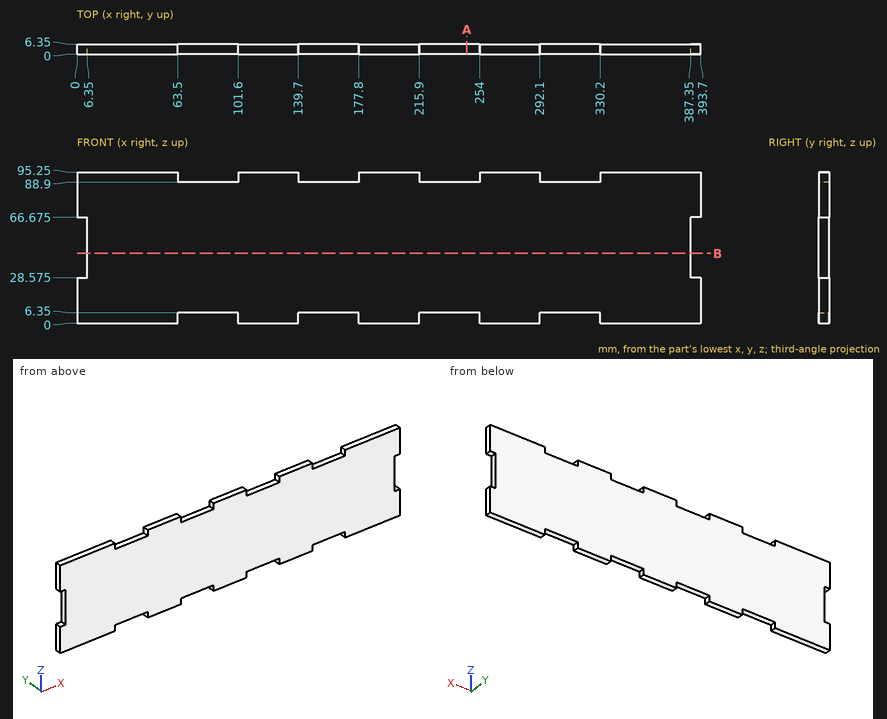
Verification items for this drawing (mm, ordinates from the low corner). Give positions to 0.01 mm unless a question says otherwise; leave off trailing zeros. Loops run counter-clockwise (first coordinate to the right, second up) from the corner with the lowest first, then second, coordinate; pieces in that order, holes last. Notation, with made-up numbers: M 19,49.25 L 69,49.25 A28 ccw 69,74.25 Z; hole C -31.75,31 d1. An arc over 180 degrees is marked long. Return JSON: item names as keys, results as strings. Group by question number.
1. Cross-section at B-B on z = 44. Record the boundary of the cut face in (x, y), plus the area to 3 significant figures.
2. Go/stop test with flat-tipped pins: pin 1 (3 mm diameter, centred on x = 316, y = 3, fed in from +Z); pin 2 (2 mm diameter, centred on y = 4.5, z = 56.5, fed in from +X); pin 3 (3 mm diameter, centred on x = 167, y = 3, fed in from -Z). Record where each tip stops, or that it passes through.
3. Cross-section at A-A on x = 246. Record the boundary of the cut face in (y, z), plus the area to 3 significant figures.
4. Thickness scan on L1, parallel to X at y = 3.75, z = 91.5; L2, parallel to X at y = 3, z = 31.5; L3, parallel to Z at x = 143, y = 5.5. Record the ranges inside material, lowest first.
Return value:
{
 "1": {"outline": "M 6.35,0 L 387.35,0 L 387.35,6.35 L 6.35,6.35 Z", "area": "2,420 mm^2"},
 "2": {"pin 1": "z = 88.9", "pin 2": "x = 387.35", "pin 3": "z = 6.35"},
 "3": {"outline": "M 0,6.35 L 6.35,6.35 L 6.35,88.9 L 0,88.9 Z", "area": "524 mm^2"},
 "4": {"L1": "0 to 63.5, 101.6 to 139.7, 177.8 to 215.9, 254 to 292.1, 330.2 to 393.7", "L2": "6.35 to 387.35", "L3": "6.35 to 88.9"}
}
